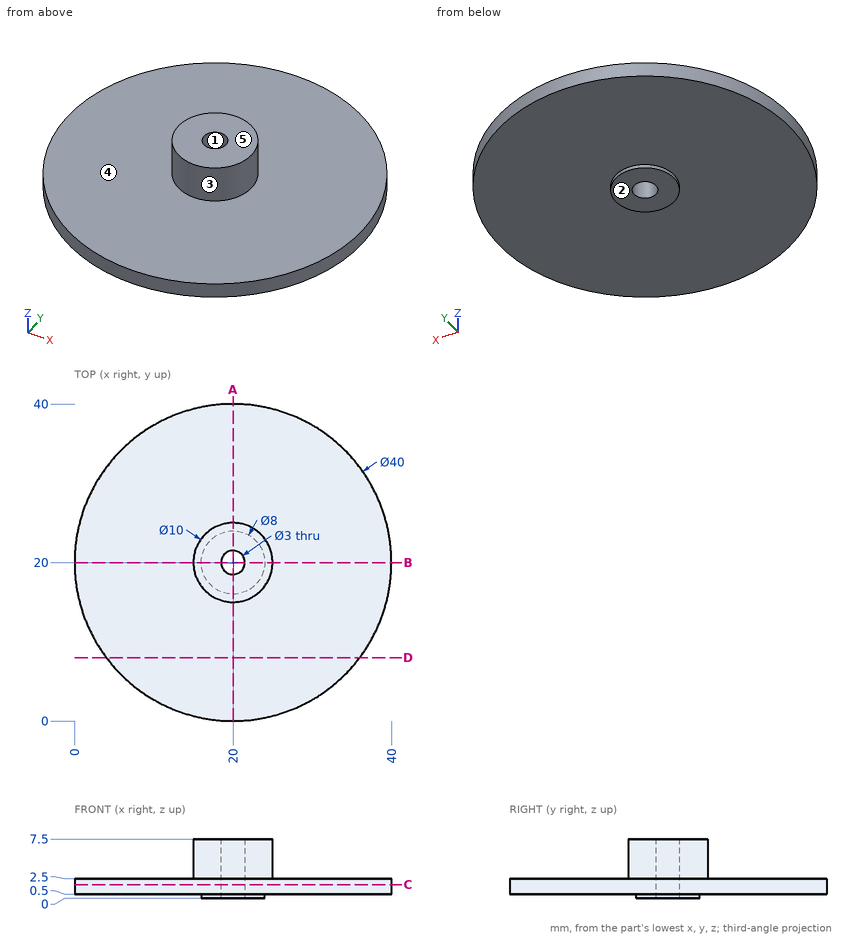
Geometry: see drawing. Coordinates: mm, zero at the bounding-box minimum. A direction names the side the tool comes from. Coordinates: 2 decimals unless noted, no trailing zeros. Loops run counter-clockwise (first coordinate to the right, second up) from the corner with the lowest first, then second, coordinate; pieces in that order, holes last. Notation, with made-up numbers: (37, 87) - (53, 87) arc R28 ccw to (53, 117) - close; hole circle Ø4 at (36.25, 33). An arc over 180 degrees is marked (long way). Return JSON: item names as keys, results as strings.
Q1. Section A-A, the plane x = 20. Return loops of the section in (y, z).
Results:
{"outline": "(0, 0.5) - (16, 0.5) - (16, 0) - (18.5, 0) - (18.5, 7.5) - (15, 7.5) - (15, 2.5) - (0, 2.5) - close; (21.5, 0) - (24, 0) - (24, 0.5) - (40, 0.5) - (40, 2.5) - (25, 2.5) - (25, 7.5) - (21.5, 7.5) - close"}
Q2. Section D-D, the plane y = 8. Return loops of the section in (x, z).
Results:
{"outline": "(4, 0.5) - (36, 0.5) - (36, 2.5) - (4, 2.5) - close"}
Q3. Mould query, pull axis Y, two halves, no side actions, for the marked faces 1, 2 and 3. Classes: released by +Y, released by -Y, zero draft, split by the parting line, or undercut.
Results:
{"face 1": "undercut", "face 2": "zero draft", "face 3": "split by the parting line"}
Q4. Contact query for flat-ended pins moving along their axis: P1, Ø20, axis at x = 23.5, y = 29, coming from the -Z side; P2, Ø5, axis at x = 29, y = 26, coming from the -Z side; P3, Ø4, axis at x = 18.5, y = 28, coming from the +Z side. Output: stop coordinate, or through.
Results:
{"P1": "z = 0", "P2": "z = 0.5", "P3": "z = 2.5"}
Q5. Material intervals for line 1 along Y through (x, z) = (20, 6); line 2 along Z through (x, y) = (22, 27.5); line 3 along Y through (x, z) = (20, 2.25), sorted ascending.
Results:
{"line 1": "15 to 18.5, 21.5 to 25", "line 2": "0.5 to 2.5", "line 3": "0 to 18.5, 21.5 to 40"}
Q6. Access query for the marked faces 4 and 5. Directions: +Z, -Z, +X, -X, +Y, -Y. A direction counts if a zero-diameter tool reaches every point of the face in a straight line with its end or side. Return the directions, or none.
Results:
{"face 4": "+Z", "face 5": "+Z, +X, -X, +Y, -Y"}
Q7. Section C-C, the plane z = 1.75. Return loops of the section in (x, y).
Results:
{"outline": "circle Ø40 at (20, 20); hole circle Ø3 at (20, 20)"}
